from build123d import *

# Parameters (mm, degrees)
BOSS_EXTRUDE1_DEPTH        = 3.175
F_1_8_0_1250_DOWEL_HOLE1_D = 3.175
F_1_8_0_1250_DOWEL_HOLE2_D = 3.175


with BuildPart() as part:
    # Sketch1 → Boss-Extrude1 (new body)
    with BuildSketch(Plane(origin=(0, 0, 0), x_dir=(1, 0, 0), z_dir=(0, 1, 0))):
        with BuildLine():
            Line((-19.05, 10.16), (-19.05, 45.72))
            ThreePointArc((-19.05, 45.72), (0, 53.221284287), (19.05, 45.72))
            Line((19.05, 45.72), (19.05, 10.16))
            Line((19.05, 10.16), (19.05, 0))
            ThreePointArc((19.05, 0), (13.97, -5.08), (8.89, 0))
            Line((8.89, 0), (8.89, 3.81))
            ThreePointArc((8.89, 3.81), (7.96006403, 6.05506403), (5.715, 6.985))
            Line((5.715, 6.985), (-15.875, 6.985))
            ThreePointArc((-15.875, 6.985), (-18.12006403, 7.91493597), (-19.05, 10.16))
        make_face()
    extrude(amount=BOSS_EXTRUDE1_DEPTH)

    # 1/8 (0.1250) Dowel Hole1 (through all)
    with Locations(Plane(origin=(0, 3.175, 0), x_dir=(1, 0, 0), z_dir=(0, 1, 0))):
        with Locations((13.97, 0)):
            Hole(F_1_8_0_1250_DOWEL_HOLE1_D / 2)

    # 1/8 (0.1250) Dowel Hole2 (through all)
    with Locations(Plane(origin=(0, 3.175, 0), x_dir=(1, 0, 0), z_dir=(0, 1, 0))):
        with Locations((-16.306687583, 55.676687583)):
            Hole(F_1_8_0_1250_DOWEL_HOLE2_D / 2)


solid = part.part
Could you check a few things on this model? Use its own coordinates, in mm. A direction names the side the tool comes from. Round coordinates to 2 decimals unless told otherwise and drop trailing zeros. Write each loop counter-clockwise with the first axis right and the second up, starting at its lowest first coordinate (ties: lowest second). Pieces come first, ordered by that corner, then holes. Notation, with made-up numbers: (-2.75, 73.5) - (17.25, 73.5) arc R11 ccw to (17.25, 86.5) - close; hole circle Ø6 at (-2.75, 71.5). An arc over 180 degrees is marked (long way). Put each result on its own line as item: value. Start each with the question number.
(1) Will these pins go through, and if not, where does the flat tip stop? pin 1 (1.6 mm diameter, centred on x = -1.5, y = 1, fed in from +Z) (3 decimals); pin 2 (1 mm diameter, centred on y = 0.5, z = -3.5, fed in from -X).
(2) I want a section at B-B, the plane x = 13.97. Please give me the cut outline in (y, z) (1 decimal), plus the area to 3 significant figures.
(3) Thinking about a two-plate mould opening in Z: for faces 3 (the flat face through (-19.05, 2, -28)), 4 (the cylindrical face through (-18.095, 1.565, -7.89)), 5 (the cylindrical face through (15.23, 1.565, 0.966)), which applies, released by +Z, released by -Z, zero draft, split by the parting line, or undercut?
(4) I want a section at C-C, the plane x = -9.5. Please give me the cut outline in (y, z) (3 decimals), plus the area to 3 significant figures.
(5) I want a section at D-D, the plane x = -14. Please give me the cut outline in (y, z) (3 decimals).
(6) I need wall thicknesses on probe 1 along Z at (x, y) = (0, 1.3) (3 decimals); probe 2 along Z at (x, y) = (13.97, 1.4); probe 3 along Z at (x, y) = (13, 0.6). Which ranges of each line are inside material? Lowest first, please.
(7) For faces 1 (the flat face through (19.05, 2, -23)), 2 (the flat face through (-5, 2, -6.985)), which set-ups out of +Z, -Z, +X, -X, +Y, -Y let a thin tool reach every point of the face, with its end or its side?
Here are the results:
1. pin 1: stops at z = -6.985
1. pin 2: stops at x = 8.88
2. outline: (0, -49.5) - (3.2, -49.5) - (3.2, -1.6) - (0, -1.6) - close; (0, 1.6) - (3.2, 1.6) - (3.2, 5.1) - (0, 5.1) - close
2. area: 163 mm^2
3. face 3: zero draft
3. face 4: released by +Z
3. face 5: undercut
4. outline: (0, -51.557) - (3.175, -51.557) - (3.175, -6.985) - (0, -6.985) - close
4. area: 142 mm^2
5. outline: (0, -49.461) - (3.175, -49.461) - (3.175, -6.985) - (0, -6.985) - close
6. probe 1: z = -53.221 to -6.985
6. probe 2: z = -49.48 to -1.59, 1.59 to 5.08
6. probe 3: z = -50.01 to -1.26, 1.26 to 4.99
7. face 1: +Z, -Z, +X, +Y, -Y
7. face 2: +Z, -X, +Y, -Y
